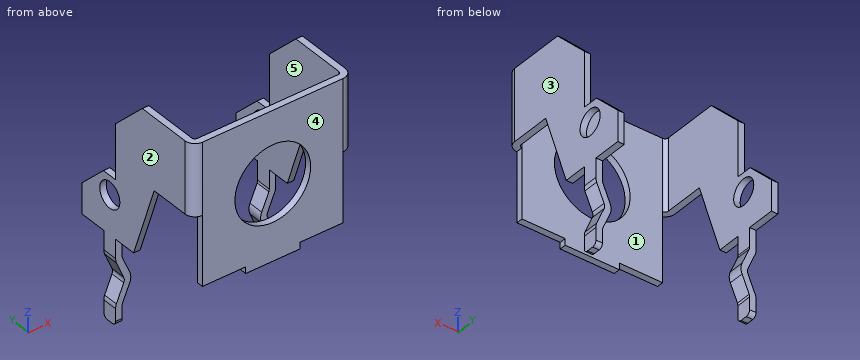
```python
from build123d import *

# Parameters (mm, degrees)
PAD_DEPTH       = 3.7
POCKET_DEPTH    = 10.701
POCKET001_DEPTH = 1
POCKET002_DEPTH = 1
SKETCH004_R     = 0.6
POCKET003_DEPTH = 7.401
FILLET_R        = 0.45
SKETCH005_R     = 1.75
POCKET004_DEPTH = 6.601


with BuildPart() as part:
    # Sketch → Pad (new body, symmetric)
    with BuildSketch(Plane.YZ):
        with BuildLine():
            Line((-4.95, 0), (-4.95, 6.8))
            Line((-4.95, 6.8), (-1.94, 6.8))
            Line((-1.94, 6.8), (-0.35, 5.21))
            Line((-0.35, 5.21), (-0.35, 2.68))
            Line((-0.35, 2.68), (0.38, 2.68))
            Line((0.38, 2.68), (1.65, 1.41))
            Line((1.65, 1.41), (1.65, 0))
            Line((1.65, 0), (0.35, 0))
            Line((0.35, 0), (0.35, -3.7))
            ThreePointArc((0.15, -3.9), (0.291421, -3.841421), (0.35, -3.7))
            Line((0.15, -3.9), (-0.15, -3.9))
            ThreePointArc((-0.35, -3.7), (-0.291421, -3.841421), (-0.15, -3.9))
            Line((-0.35, -3.7), (-0.35, 0))
            Line((-0.35, 0), (-1.425, 0))
            Line((-1.425, 0), (-2.65, 3.5))
            Line((-2.65, 3.5), (-4.65, 3.5))
            Line((-4.65, 3.5), (-4.65, 0))
            Line((-4.65, 0), (-4.95, 0))
        make_face()
    extrude(amount=PAD_DEPTH, both=True)

    # Sketch001 (on Face8 of Pad) → Pocket (cut, through all)
    with BuildSketch(Plane(origin=(0, 0, 6.8), x_dir=(0, -1, 0), z_dir=(0, 0, 1))):
        with BuildLine():
            Line((-2.38, -3.4), (-0.35, -3.4))
            Line((-0.35, -3.4), (-0.35, -3))
            Line((-0.35, -3), (0.35, -3))
            Line((0.35, -3), (0.35, -3.4))
            Line((0.35, -3.4), (4.5, -3.4))
            ThreePointArc((4.5, -3.4), (4.606066, -3.356066), (4.65, -3.25))
            Line((4.65, -3.25), (4.65, 3.25))
            ThreePointArc((4.65, 3.25), (4.606066, 3.356066), (4.5, 3.4))
            Line((4.5, 3.4), (0.35, 3.4))
            Line((0.35, 3.4), (0.35, 3))
            Line((0.35, 3), (-0.38, 3))
            Line((-0.38, 3), (-0.38, 3.4))
            Line((-0.38, 3.4), (-2.38, 3.4))
            Line((-2.38, 3.4), (-2.38, -3.4))
        make_face()
    extrude(amount=-POCKET_DEPTH, mode=Mode.SUBTRACT)

    # Sketch002 (on Face33 of Pocket) → Pocket001 (cut, symmetric)
    with BuildSketch(Plane.ZX.offset(0.35)):
        with BuildLine():
            Line((-4.2, 3.4), (-3.13, 3.4))
            ThreePointArc((-3.013051, 3.382522), (-3.070876, 3.395606), (-3.13, 3.4))
            Line((-3.013051, 3.382522), (-2.244042, 3.051873))
            ThreePointArc((-2.244042, 3.051873), (-2, 3), (-1.755958, 3.051873))
            Line((-1.755958, 3.051873), (-0.986949, 3.382522))
            ThreePointArc((-0.87, 3.4), (-0.929124, 3.395606), (-0.986949, 3.382522))
            Line((-0.87, 3.4), (2.68, 3.4))
            Line((2.68, 3.4), (2.98, 3.4))
            Line((2.98, 3.4), (2.98, 2.7))
            Line((2.98, 2.7), (-4.2, 2.7))
            Line((-4.2, 2.7), (-4.2, 3))
            Line((-4.2, 3), (-4.2, 3.4))
        make_face()
        with BuildLine():
            ThreePointArc((-2.92534, 3.669413), (-3.026533, 3.692311), (-3.13, 3.7))
            Line((-3.13, 3.7), (-3.13, 3.9))
            Line((-3.13, 3.9), (-0.87, 3.9))
            Line((-0.87, 3.9), (-0.87, 3.7))
            ThreePointArc((-0.87, 3.7), (-0.973467, 3.692311), (-1.07466, 3.669413))
            Line((-1.877979, 3.325936), (-1.07466, 3.669413))
            ThreePointArc((-2.122021, 3.325936), (-2, 3.3), (-1.877979, 3.325936))
            Line((-2.92534, 3.669413), (-2.122021, 3.325936))
        make_face()
    pocket001 = extrude(amount=POCKET001_DEPTH, both=True, mode=Mode.SUBTRACT)

    # Mirrored: Pocket001 across Sketch002 H_Axis
    add(pocket001.mirror(Plane(origin=(0, 0.35, 0), x_dir=(0, 1, 0), z_dir=(1, 0, 0))), mode=Mode.SUBTRACT)

    # Sketch003 (on Face26 of Mirrored) → Pocket002 (cut)
    with BuildSketch(Plane(origin=(0, -4.95, 0), x_dir=(0, 0, -1), z_dir=(0, -1, 0))):
        Polygon((0, -1.25), (-0.3, -1.25), (-0.3, -3.25), (-3.5, -3.25), (-3.5, -3.7), (-3.5, -4.2), (0.5, -4.2), (0.5, -1.25), align=None)
    pocket002 = extrude(amount=-POCKET002_DEPTH, mode=Mode.SUBTRACT)

    # Mirrored001: Pocket002 across Sketch003 H_Axis
    add(pocket002.mirror(Plane(origin=(0, -4.95, 0), x_dir=(0, -1, 0), z_dir=(1, 0, 0))), mode=Mode.SUBTRACT)

    # Sketch004 (on Face9 of Mirrored001) → Pocket003 (cut, through all)
    with BuildSketch(Plane(origin=(-3.7, 0, 0), x_dir=(0, 1, 0), z_dir=(-1, 0, 0))):
        with Locations((0, -1.8)):
            Circle(SKETCH004_R)
    extrude(amount=-POCKET003_DEPTH, mode=Mode.SUBTRACT)

    # Fillet
    fillet_edges = [part.edges().sort_by_distance(p)[0] for p in [
        (-3.7, -4.95, 5.15),
        (3.7, -4.95, 5.15),
    ]]
    fillet(fillet_edges, radius=FILLET_R)

    # Sketch005 (on Face20 of Fillet) → Pocket004 (cut, through all)
    with BuildSketch(Plane.XZ.offset(4.95)):
        with Locations((0, 3.5)):
            Circle(SKETCH005_R)
    extrude(amount=-POCKET004_DEPTH, mode=Mode.SUBTRACT)


solid = part.part
```
The listing builds one solid part. Answer for the finished solid, in the listing's coordinates (mm). Face numbers are marked on the shaded views. A direction names the side the tool comes from. Round coordinates to 2 decimals unless told otherwise and drop trailing zeros. Loops run counter-clockwise (first coordinate to the right, second up) from the corner with the lowest first, then second, coordinate; pieces in that order, holes last.
Q1. Given pin 1 Ø0.6 at (x, z) = (3.5, -2.5) entering from +Y, flat-ended and moving along its own axis, determine where the tip first touches the part or whether it passes through.
Q2. Section D-D, the plane x = -2.5 is taken. Determine the outline of the cut face in (y, z).
Q3. Section B-B, the plane x = 0 is taken. Determine the outline of the cut face in (y, z).
Q4. Which of the six approach directions +Z, -Z, +X, -X, +Y, -Y give full straight-line access (tool end or side, diameter ignored) to the marked faces 1 and 2?
Q5. Section A-A, the plane y = -4 is taken. Determine the outline of the cut face in (x, z), then the cut area to 3 significant figures.
Q6. Section C-C, the plane z = 4.75 is taken. Determine the outline of the cut face in (x, y), then the cut area to 3 significant figures.
Q7. For a pull along X with two mould halves and no side action, classify the marked faces 3, 4 and 5 as released by +X, released by -X, zero draft, split by the parting line, or undercut.
Q8. Find the intervals of material crossed by line 1 (X direction, y = -0.5, z = 4.75); line 2 (Z direction, x = 0, y = -4.7); line 3 (Z direction, x = 3.55, y = 0), in increasing order.
Completed:
1. pin 1: stops at y = 0.35
2. outline: (-4.95, 0.3) - (-4.65, 0.3) - (-4.65, 6.8) - (-4.95, 6.8) - close
3. outline: (-4.95, 0) - (-4.65, 0) - (-4.65, 1.75) - (-4.95, 1.75) - close; (-4.95, 5.25) - (-4.65, 5.25) - (-4.65, 6.8) - (-4.95, 6.8) - close
4. face 1: +Z, -Z, +Y
4. face 2: +Z, -Z, -X, +Y, -Y
5. outline: (-3.7, 3.5) - (-3.4, 3.5) - (-3.4, 6.8) - (-3.7, 6.8) - close; (3.4, 3.5) - (3.7, 3.5) - (3.7, 6.8) - (3.4, 6.8) - close
5. area: 1.98 mm2
6. outline: (-3.7, -4.5) arc R0.45 ccw to (-3.25, -4.95) - (-1.22, -4.95) - (-1.22, -4.65) - (-3.25, -4.65) arc R0.15 cw to (-3.4, -4.5) - (-3.4, -0.35) - (-3.7, -0.35) - close; (1.22, -4.95) - (3.25, -4.95) arc R0.45 ccw to (3.7, -4.5) - (3.7, -0.35) - (3.4, -0.35) - (3.4, -4.5) arc R0.15 cw to (3.25, -4.65) - (1.22, -4.65) - close
6. area: 3.99 mm2
7. face 3: released by +X
7. face 4: zero draft
7. face 5: undercut
8. line 1: x = -3.7 to -3.4, 3.4 to 3.7
8. line 2: z = 0 to 1.75, 5.25 to 6.8
8. line 3: z = -3.9 to -2.65, -1.35 to 1.2, 2.4 to 2.68
